Geometry check sheet. Reference: the model listing, model coordinates, mm. Face numbers are marked on the shaded views. A direction names the side the tool comes from. Give positions to 0.01 mm unless a question says otherwise; leave off trailing zeros. Loops run counter-clockwise (first coordinate to the right, second up) from the corner with the lowest first, then second, coordinate; pieces in that order, holes last. Notation, with made-up numbers: (37, 0.25) -> (43, 0.25) arc R14 cw to (43, 12.25) -> close; hole circle Ø9 at (7.5, 55.5). An arc over 180 degrees is marked (long way). Write item = value, one per line.
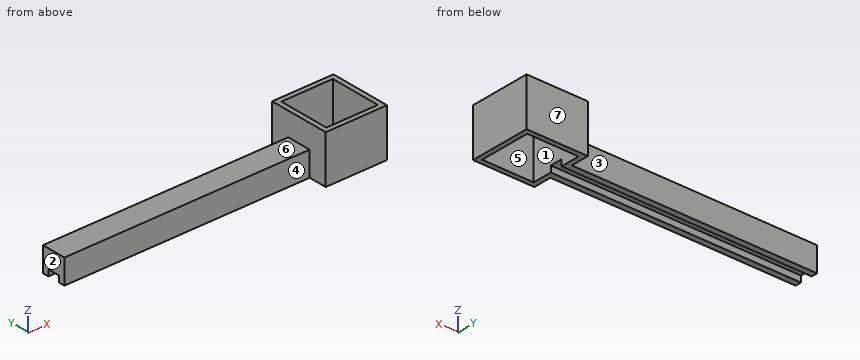
```python
from build123d import *

# Parameters (mm, degrees)
ESQUISSE1_W             = 200
ESQUISSE1_H             = 20
ESQUISSE1_W_2           = 42
ESQUISSE1_H_2           = 42
BOSS_EXTRU_1_DEPTH      = 39
ESQUISSE2_W             = 200
ESQUISSE2_H             = 20
ENL_V_MAT_EXTRU_1_DEPTH = 19
ESQUISSE3_W             = 204
ESQUISSE3_H             = 10
ENL_V_MAT_EXTRU_3_DEPTH = 5


with BuildPart() as part:
    # Esquisse1 → Boss.-Extru.1 (new body)
    with BuildSketch(Plane.XY):
        with Locations((100, -10)):
            Rectangle(ESQUISSE1_W, ESQUISSE1_H)
        Polygon((200, 15), (200, 0), (200, -20), (200, -35), (250, -35), (250, 15), align=None)
        with Locations((225, -10)):
            Rectangle(ESQUISSE1_W_2, ESQUISSE1_H_2, mode=Mode.SUBTRACT)
    extrude(amount=BOSS_EXTRU_1_DEPTH)

    # Esquisse2 → Enlèv. mat.-Extru.1 (cut)
    with BuildSketch(Plane.XY.offset(39)):
        with Locations((100, -10)):
            Rectangle(ESQUISSE2_W, ESQUISSE2_H)
    extrude(amount=-ENL_V_MAT_EXTRU_1_DEPTH, mode=Mode.SUBTRACT)

    # Esquisse3 → Enlèv. mat.-Extru.3 (cut)
    with BuildSketch(Plane(origin=(0, 0, 0), x_dir=(-1, 0, 0), z_dir=(0, 0, -1))):
        with Locations((-102, -10)):
            Rectangle(ESQUISSE3_W, ESQUISSE3_H)
    extrude(amount=-ENL_V_MAT_EXTRU_3_DEPTH, mode=Mode.SUBTRACT)


solid = part.part
```
Item 1: Draft check along X on the marked faces 1, 2 and 3. Enter one of: +X half, -X half, draft (parallel to the pull), parting line (faces both ways), or undercut.
Answer:
face_1 = undercut
face_2 = -X half
face_3 = draft
Item 2: Tool access check on the marked faces 4, 5, 6 and 7. Record the directions out of +Z, -Z, +X, -X, +Y, -Y that give a thin tool (end or side, any length) a straight path to the whole face; none if there is none.
Answer:
face_4 = +Z, -Z, -X, -Y
face_5 = +Z, -Z
face_6 = +Z, -X, +Y, -Y
face_7 = +Z, -Z, +X, -X, +Y
Item 3: Section check C-C, the plane x = 57. Record the cut outline in (y, z).
Answer:
outline = (-20, 0) -> (-15, 0) -> (-15, 5) -> (-5, 5) -> (-5, 0) -> (0, 0) -> (0, 20) -> (-20, 20) -> close
Item 4: Section check A-A, the plane z = 14.5. Record the cut outline in (x, y), plus the area to 3 significant figures.
Answer:
outline = (0, -20) -> (200, -20) -> (200, -35) -> (250, -35) -> (250, 15) -> (200, 15) -> (200, 0) -> (0, 0) -> close; hole (204, -31) -> (246, -31) -> (246, 11) -> (204, 11) -> close
area = 4,740 mm^2
Item 5: Thickness scan on L1, parallel to X at y = -16, z = 5.5; L2, parallel to X at y = -0.5, z = 33; L3, parallel to Y at x = 224.5, z = 36.5. Record the ranges inside material, lowest first. Write a range as [from, to].
Answer:
L1 = [0, 204], [246, 250]
L2 = [200, 204], [246, 250]
L3 = [-35, -31], [11, 15]
Item 6: Section check D-D, the plane z = 25. Record the cut outline in (x, y), plus the area to 3 significant figures.
Answer:
outline = (200, -35) -> (250, -35) -> (250, 15) -> (200, 15) -> close; hole (204, -31) -> (246, -31) -> (246, 11) -> (204, 11) -> close
area = 736 mm^2
Item 7: Gauge pin test, flat ends, axial feed: pin 1 (3 mm diameter, centred on x = 53, y = -7.5, fed in from -Z); pin 2 (22 mm diameter, centred on x = 106, y = -14, fed in from +Z); pin 3 (8 mm diameter, centred on x = 52, z = 8.5, fed in from -Y). Record the tip position at first contact, or that the pin passes through.
Answer:
pin_1 = 5
pin_2 = 20
pin_3 = -20
Item 8: Section check B-B, the plane y = -8. Record the cut outline in (x, z).
Answer:
outline = (0, 5) -> (204, 5) -> (204, 39) -> (200, 39) -> (200, 20) -> (0, 20) -> close; (246, 0) -> (250, 0) -> (250, 39) -> (246, 39) -> close
